Check sheet for the modelled part. Datum: model origin and axes. Units: mm. Coordinates: 2 decimals unless noted, no trailing zeros. Loops run counter-clockwise (first coordinate to the right, second up) from the corner with the lowest first, then second, coordinate; pieces in that order, holes last. Notation, with made-up numbers: M -37.75,3.25 L -20.75,3.25 A25 ccw -20.75,30.25 Z; hole C 46,-21.75 d4. An arc over 180 degrees is marked long. Write each question's results on one line, items separated by ' | '. Start each with the question number.
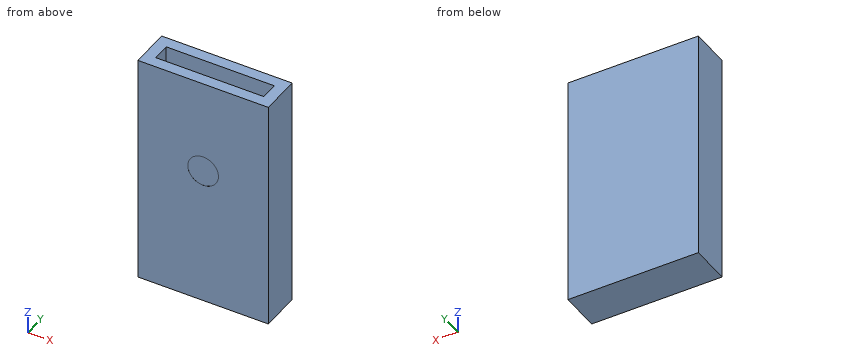
from build123d import *

# Parameters (mm, degrees)
F0_W     = 127
F0_H     = 39.0351824462
F1_DEPTH = 228.6
F2_T     = -10.8857142857
F3_R     = 14.9416499322
F4_DEPTH = 0.0762


# Not quite as in the source:
# - a length typed as a fraction of an inch, garbled in the dataset ("3 / 203.2 mm" for 3/8 in), is restored


with BuildPart() as f1:
    # F0 (on Top) → F1 (new body)
    with BuildSketch(Plane.XY):
        Rectangle(F0_W, F0_H)
    extrude(amount=F1_DEPTH)

    # F2
    f2_openings = [f1.faces().sort_by_distance(p)[0] for p in [
        (0, 0, 228.6),
    ]]
    offset(amount=F2_T, openings=f2_openings)

    # F3 (on face) → F4 (cut)
    with BuildSketch(Plane.XZ.offset(19.5175912231)):
        with Locations((0, 136.5711838007)):
            Circle(F3_R)
    extrude(amount=-F4_DEPTH, mode=Mode.SUBTRACT)


solid = f1.part
1) Section check A-A (z = 180.5). Enter the section's corners in (x, y).
2) Section check D-D (x = 0). Enter the section's corners in (y, z).
3) Thickness scan on probe 1 along Y at (x, z) = (15, 193); probe 2 along X at (y, z) = (8.5, 150); probe 3 along Z at (x, y) = (-10, -8.5). Record the ranges inside material, lowest first.
4) Section check C-C (y = 1). Enter the section's corners in (x, z).
5) Gauge pin test, flat ends, axial feed: P1, Ø15, axis at x = 7, z = 140, coming from the -Y side; P2, Ø2, axis at x = 28, y = 1.5, coming from the +Z side. Record the tip position at first contact, or that the pin passes through.
6) Section check B-B (x = 17.5). Enter the section's corners in (y, z), then the cut area to 3 significant figures.
Return value:
1) outline: M -63.5,-19.52 L 63.5,-19.52 L 63.5,19.52 L -63.5,19.52 Z; hole M -52.61,-8.63 L 52.61,-8.63 L 52.61,8.63 L -52.61,8.63 Z
2) outline: M -19.52,0 L 19.52,0 L 19.52,228.6 L 8.63,228.6 L 8.63,10.89 L -8.63,10.89 L -8.63,228.6 L -19.52,228.6 L -19.52,151.51 L -19.44,151.51 L -19.44,121.63 L -19.52,121.63 Z
3) probe 1: y = -19.52 to -8.63, 8.63 to 19.52 | probe 2: x = -63.5 to -52.61, 52.61 to 63.5 | probe 3: z = 0 to 10.89
4) outline: M -63.5,0 L 63.5,0 L 63.5,228.6 L 52.61,228.6 L 52.61,10.89 L -52.61,10.89 L -52.61,228.6 L -63.5,228.6 Z
5) P1: stops at y = -19.52 | P2: stops at z = 10.89
6) outline: M -19.52,0 L 19.52,0 L 19.52,228.6 L 8.63,228.6 L 8.63,10.89 L -8.63,10.89 L -8.63,228.6 L -19.52,228.6 Z | area: 5,160 mm2
